```python
from build123d import *

# Parameters (mm, degrees)
EXTRUDE_1_DEPTH     = 36
SKETCH_2_R          = 1.75
CUT_EXTRUDE_1_DEPTH = 35
FILLET_1_R          = 1.5
FILLET_2_R          = 3
CUT_EXTRUDE_5_DEPTH = 50
SKETCH_5_W          = 24
SKETCH_5_H          = 86
SKETCH_5_R          = 5.25
EXTRUDE_2_DEPTH     = 1.5
SKETCH_6_W          = 2
SKETCH_6_H          = 6.336440046
CUT_EXTRUDE_6_DEPTH = 3.5
FILLET_3_R          = 1.5
FILLET_4_R          = 3
CHAMFER_1_SIZE      = 2
SKETCH_7_W          = 36
SKETCH_7_H          = 1.5
CUT_EXTRUDE_7_DEPTH = 4


with BuildPart() as part:
    # Эскиз1 → Вытянуть1 (new body)
    with BuildSketch(Plane.XY):
        Polygon((-32, 43.5), (0, 43.5), (0, 0), (36, 0), (36, 43.5), (60, 43.5), (60, 42), (37.5, 42), (37.5, -1.5), (-1.5, -1.5), (-1.5, 42), (-32, 42), align=None)
    extrude(amount=EXTRUDE_1_DEPTH)

    # Эскиз2 → Вырез-Вытянуть1 (cut)
    with BuildSketch(Plane(origin=(0, 43.5, 0), x_dir=(-1, 0, 0), z_dir=(0, 1, 0))):
        with Locations(Location((22, 5, 0), (0, 0, 90))):
            Circle(SKETCH_2_R)
        with Locations(Location((22, 31, 0), (0, 0, 90))):
            Circle(SKETCH_2_R)
    extrude(amount=-CUT_EXTRUDE_1_DEPTH, mode=Mode.SUBTRACT)

    # Скругление1
    fillet_1_edges = [part.edges().sort_by_distance(p)[0] for p in [
        (0, 0, 18),
        (36, 0, 18),
        (-1.5, 42, 18),
    ]]
    fillet(fillet_1_edges, radius=FILLET_1_R)

    # Скругление2
    fillet_2_edges = [part.edges().sort_by_distance(p)[0] for p in [
        (0, 43.5, 18),
        (37.5, -1.5, 18),
        (-1.5, -1.5, 18),
    ]]
    fillet(fillet_2_edges, radius=FILLET_2_R)

    # Эскиз4 → Вырез-Вытянуть5 (cut)
    with BuildSketch(Plane.ZY.offset(1.5)):
        Polygon((36, 0), (30.401923789, -1.5), (5.598076211, -1.5), (0, 0), (0, -9.726752533), (36, -8.93099636), align=None)
    extrude(amount=-CUT_EXTRUDE_5_DEPTH, mode=Mode.SUBTRACT)

    # Эскиз5 → Вытянуть2 (add)
    with BuildSketch(Plane(origin=(0, 43.5, 0), x_dir=(-1, 0, 0), z_dir=(0, 1, 0))):
        with Locations((-48, 18)):
            Rectangle(SKETCH_5_W, SKETCH_5_H)
        with Locations(Location((-48, -15, 0), (0, 0, 90))):
            Circle(SKETCH_5_R, mode=Mode.SUBTRACT)
        with Locations(Location((-48, 51, 0), (0, 0, 270))):
            Circle(SKETCH_5_R, mode=Mode.SUBTRACT)
    extrude(amount=-EXTRUDE_2_DEPTH)

    # Эскиз6 → Вырез-Вытянуть6 (cut)
    with BuildSketch(Plane.ZY.offset(-36)):
        with Locations((37, 42.938728947)):
            Rectangle(SKETCH_6_W, SKETCH_6_H)
        with Locations((-1, 42.938728947)):
            Rectangle(SKETCH_6_W, SKETCH_6_H)
    extrude(amount=-CUT_EXTRUDE_6_DEPTH, mode=Mode.SUBTRACT)

    # Скругление3
    fillet_3_edges = [part.edges().sort_by_distance(p)[0] for p in [
        (37.5, 42, 18),
    ]]
    fillet(fillet_3_edges, radius=FILLET_3_R)

    # Скругление4
    fillet_4_edges = [part.edges().sort_by_distance(p)[0] for p in [
        (36, 43.5, 18),
    ]]
    fillet(fillet_4_edges, radius=FILLET_4_R)

    # Фаска1
    chamfer_1_edges = [part.edges().sort_by_distance(p)[0] for p in [
        (36, 42.75, 61),
        (36, 42.75, -25),
        (60, 42.75, -25),
        (60, 42.75, 61),
    ]]
    chamfer(chamfer_1_edges, length=CHAMFER_1_SIZE)

    # Эскиз7 → Вырез-Вытянуть7 (cut)
    with BuildSketch(Plane.ZY.offset(32)):
        with Locations((18, 42.75)):
            Rectangle(SKETCH_7_W, SKETCH_7_H)
    extrude(amount=-CUT_EXTRUDE_7_DEPTH, mode=Mode.SUBTRACT)


solid = part.part
```
Geometry check sheet. Reference: the model listing, model coordinates, mm. A direction names the side the tool comes from. Give positions to 0.01 mm unless a question says otherwise; leave off trailing zeros. Write each loop counter-clockwise with the first axis right and the second up, starting at its lowest first coordinate (ties: lowest second). Pieces come first, ordered by that corner, then holes.
1) Section check B-B, the plane x = -22. Record the boundary of the cut face in (y, z).
2) Access from +Z, -Z, +X, -X, +Y, -Y to the whole of each face (thin tool, end or side, straight path). Record for faces 1 (the flat face through (-1, 28, 36)), 2 (the flat face through (-16, 43.5, 18)), 3 (the flat face through (-1, 28, 0)), 4 (the cylindrical face through (-0.64, -0.6, 18.25)), 5 (the flat face through (18, 0, 18)).
3) Section check D-D, the plane z = 8.5. Record the boundary of the cut face in (x, y).
4) Section check C-C, the plane y = 29. Record the boundary of the cut face in (x, z).
5) Section check A-A, the plane z = 51. Record the boundary of the cut face in (x, y).
6) Material ranges on L1, parallel to X at y = 43.1, z = -15; L2, parallel to X at y = 5.5, z = 7; L3, parallel to X at y = 42.6, z = 5, recorded low to high.
7) Release check for a two-part mould opening along X. For faces 6 (the flat face through (-1.5, 21, 18)), 7 (the cylindrical face through (44.45, 42.76, 54.87)), 8 (the flat face through (48, 43.5, 19)) record: pulls with the +X half, pulls with the -X half, needs draft (parallel to the pull), parting line crosses it, or undercut.
8) Gauge pin test, flat ends, axial feed: pin 1 (1.6 mm diameter, centred on y = 43, z = 44, fed in from -X); pin 2 (7 mm diameter, centred on x = 53, z = 11.5, fed in from -Y); pin 3 (8 mm diameter, centred on x = 26, z = -2, fed in from +Y). Record the tip position at first contact, or that the pin passes through.
Computed:
1. outline: (42, 0) - (43.5, 0) - (43.5, 3.25) - (42, 3.25) - close; (42, 6.75) - (43.5, 6.75) - (43.5, 29.25) - (42, 29.25) - close; (42, 32.75) - (43.5, 32.75) - (43.5, 36) - (42, 36) - close
2. face 1: +Z, -X, +Y, -Y
2. face 2: +Z, -Z, +X, -X, +Y
2. face 3: -Z, -X, +Y, -Y
2. face 4: +Z, -Z, -X, -Y
2. face 5: +Z, -Z, +Y
3. outline: (-28, 42) - (-3, 42) arc R1.5 cw to (-1.5, 40.5) - (-1.5, 1.5) arc R3 ccw to (1.5, -1.5) - (34.5, -1.5) arc R3 ccw to (37.5, 1.5) - (37.5, 40.5) arc R1.5 cw to (39, 42) - (60, 42) - (60, 43.5) - (39, 43.5) arc R3 ccw to (36, 40.5) - (36, 1.5) arc R1.5 cw to (34.5, 0) - (1.5, 0) arc R1.5 cw to (0, 1.5) - (0, 40.5) arc R3 ccw to (-3, 43.5) - (-28, 43.5) - close
4. outline: (-1.5, 0) - (0, 0) - (0, 36) - (-1.5, 36) - close; (36, 0) - (37.5, 0) - (37.5, 36) - (36, 36) - close
5. outline: (36, 42) - (42.75, 42) - (42.75, 43.5) - (36, 43.5) - close; (53.25, 42) - (60, 42) - (60, 43.5) - (53.25, 43.5) - close
6. L1: x = 36 to 42.75, 53.25 to 60
6. L2: x = -1.5 to 0, 36 to 37.5
6. L3: x = -28 to -23.75, -20.25 to -0.86, 36.86 to 60
7. face 6: pulls with the -X half
7. face 7: undercut
7. face 8: needs draft
8. pin 1: stops at x = 36
8. pin 2: stops at y = 42
8. pin 3: stops at y = 0
